For this review, take the finished solid that the model builds, in its own axes (mm). Face numbers are marked on the shaded views. Coordinates: 2 decimals unless noted, no trailing zeros. One line per item, written item: value. Start each with the question number.
1) Add section A-A (y = 7). State how many separate pieces and enclosed holes the cut face has, and give its area (3 significant figures).
2) Mouldability with a two-part tool opening along Z and no side actions: class the marked faces 1 and 2 as released by +Z, released by -Z, zero draft, split by the parting line, or undercut.
3) For probe 1 along Y at (x, z) = (117, -112); probe 2 along X at (y, z) = (6, -137), list the stretches that pass through material, from the lowest coordinate up. Write a range as from..to.
4) For pin 1 Ø0.9 at (y, z) = (4, -22.5) entering from +X; pin 2 Ø3 at (y, z) = (6, -78) entering from -X; pin 3 Ø1.5 at (x, y) = (28, 5.5) entering from +Z; pin 4 Ø1 at (y, z) = (4, -91.5) entering from -X, all flat-tipped, find the tip position at first contact; note any pin that passes through.
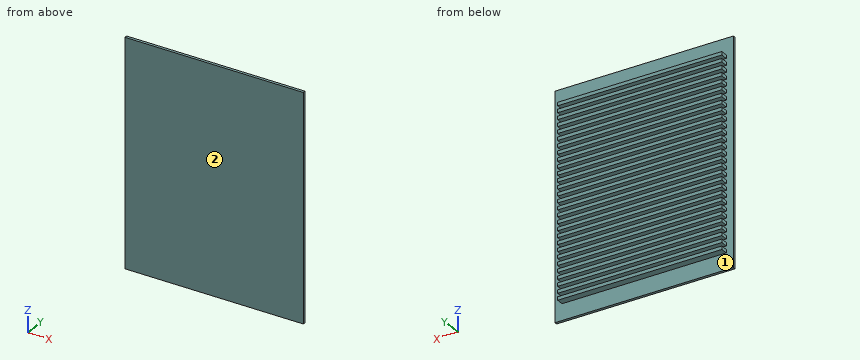
from build123d import *

# Parameters (mm, degrees)
SKETCH1_W           = 160.782
SKETCH1_H           = 203.2
BOSS_EXTRUDE1_DEPTH = 2.413
SKETCH2_W           = 148.082
SKETCH2_H           = 3.048
BOSS_EXTRUDE2_DEPTH = 6.35


with BuildPart() as part:
    # Sketch1 → Boss-Extrude1 (new body)
    with BuildSketch(Plane(origin=(0, 0, 0), x_dir=(1, 0, 0), z_dir=(0, 1, 0))):
        with Locations((80.391, 101.6)):
            Rectangle(SKETCH1_W, SKETCH1_H)
    extrude(amount=BOSS_EXTRUDE1_DEPTH)

    # Sketch2 → Boss-Extrude2 (add)
    with BuildSketch(Plane(origin=(0, 2.413, 0), x_dir=(1, 0, 0), z_dir=(0, 1, 0))):
        with Locations((80.391, 180.848)):
            Rectangle(SKETCH2_W, SKETCH2_H)
        with Locations((80.391, 186.944)):
            Rectangle(SKETCH2_W, SKETCH2_H)
        with Locations((80.391, 174.752)):
            Rectangle(SKETCH2_W, SKETCH2_H)
        with Locations((80.391, 168.656)):
            Rectangle(SKETCH2_W, SKETCH2_H)
        with Locations((80.391, 162.56)):
            Rectangle(SKETCH2_W, SKETCH2_H)
        with Locations((80.391, 156.464)):
            Rectangle(SKETCH2_W, SKETCH2_H)
        with Locations((80.391, 150.368)):
            Rectangle(SKETCH2_W, SKETCH2_H)
        with Locations((80.391, 144.272)):
            Rectangle(SKETCH2_W, SKETCH2_H)
        with Locations((80.391, 138.176)):
            Rectangle(SKETCH2_W, SKETCH2_H)
        with Locations((80.391, 132.08)):
            Rectangle(SKETCH2_W, SKETCH2_H)
        with Locations((80.391, 125.984)):
            Rectangle(SKETCH2_W, SKETCH2_H)
        with Locations((80.391, 119.888)):
            Rectangle(SKETCH2_W, SKETCH2_H)
        with Locations((80.391, 113.792)):
            Rectangle(SKETCH2_W, SKETCH2_H)
        with Locations((80.391, 107.696)):
            Rectangle(SKETCH2_W, SKETCH2_H)
        with Locations((80.391, 101.6)):
            Rectangle(SKETCH2_W, SKETCH2_H)
        with Locations((80.391, 95.504)):
            Rectangle(SKETCH2_W, SKETCH2_H)
        with Locations((80.391, 89.408)):
            Rectangle(SKETCH2_W, SKETCH2_H)
        with Locations((80.391, 83.312)):
            Rectangle(SKETCH2_W, SKETCH2_H)
        with Locations((80.391, 77.216)):
            Rectangle(SKETCH2_W, SKETCH2_H)
        with Locations((80.391, 71.12)):
            Rectangle(SKETCH2_W, SKETCH2_H)
        with Locations((80.391, 65.024)):
            Rectangle(SKETCH2_W, SKETCH2_H)
        with Locations((80.391, 58.928)):
            Rectangle(SKETCH2_W, SKETCH2_H)
        with Locations((80.391, 52.832)):
            Rectangle(SKETCH2_W, SKETCH2_H)
        with Locations((80.391, 46.736)):
            Rectangle(SKETCH2_W, SKETCH2_H)
        with Locations((80.391, 40.64)):
            Rectangle(SKETCH2_W, SKETCH2_H)
        with Locations((80.391, 34.544)):
            Rectangle(SKETCH2_W, SKETCH2_H)
        with Locations((80.391, 28.448)):
            Rectangle(SKETCH2_W, SKETCH2_H)
        with Locations((80.391, 22.352)):
            Rectangle(SKETCH2_W, SKETCH2_H)
        with Locations((80.391, 16.256)):
            Rectangle(SKETCH2_W, SKETCH2_H)
    extrude(amount=BOSS_EXTRUDE2_DEPTH)


solid = part.part
Numbers:
1. separate pieces: 29
1. enclosed holes: 0
1. area: 13,100 mm²
2. face 1: undercut
2. face 2: zero draft
3. probe 1: 0..2.41
3. probe 2: 6.35..154.43
4. pin 1: x = 154.43
4. pin 2: x = 6.35
4. pin 3: z = -14.73
4. pin 4: through
